CAD build for the part. Positions are in the model's coordinates, mm. A direction names the side the tool comes from. Give positions to 0.01 mm unless a question says otherwise; leave off trailing zeros. Loops run counter-clockwise (first coordinate to the right, second up) from the corner with the lowest first, then second, coordinate; pieces in that order, holes last.
```python
from build123d import *

# Parameters (mm, degrees)
F0_W     = 56
F0_H     = 50
F0_R     = 1.65
F0_R_2   = 23
F0_R_3   = 21.5
F1_DEPTH = 28
F2_R     = 21.5
F3_DEPTH = 25
F4_R     = 1.65
F5_DEPTH = 28.001
F7_DEPTH = 25
F6_R     = 23
F6_R_2   = 21.5
F8_DEPTH = 25


with BuildPart() as f1:
    # F0 (on Front) → F1 (new body)
    with BuildSketch(Plane.XZ):
        Rectangle(F0_W, F0_H)
        with Locations((23, -20)):
            Circle(F0_R, mode=Mode.SUBTRACT)
        with Locations((-23, 20)):
            Circle(F0_R, mode=Mode.SUBTRACT)
        Circle(F0_R_2, mode=Mode.SUBTRACT)
        Circle(F0_R_2)
        Circle(F0_R_3, mode=Mode.SUBTRACT)
        Circle(F0_R_3)
        with Locations((23, -20)):
            Circle(F0_R)
        with Locations((-23, 20)):
            Circle(F0_R)
    extrude(amount=F1_DEPTH)

    # F2 (on face) → F3 (cut)
    with BuildSketch(Plane.XZ.offset(28)):
        Circle(F2_R)
    extrude(amount=-F3_DEPTH, mode=Mode.SUBTRACT)

    # F4 (on face) → F5 (cut, through all)
    with BuildSketch(Plane.XZ.offset(28)):
        with Locations((-23, 20)):
            Circle(F4_R)
        with Locations((23, -20)):
            Circle(F4_R)
    extrude(amount=-F5_DEPTH, mode=Mode.SUBTRACT)

    # F7 (cut): a face of the model
    f7_faces = [f1.faces().sort_by_distance(p)[0] for p in [
        (0, -28, -24.2492670248),
    ]]
    extrude(f7_faces, amount=-F7_DEPTH, mode=Mode.SUBTRACT)

    # F6 (on face) → F8 (join)
    with BuildSketch(Plane.XZ.offset(3)):
        Circle(F6_R)
        Circle(F6_R_2, mode=Mode.SUBTRACT)
    extrude(amount=F8_DEPTH)


solid = f1.part
```
1. Saw through at B-B, the plane y = -4. List the corners of the cut face in (x, z), and give its area (3 significant figures).
Responses:
outline: circle Ø46 at (0, 0); hole circle Ø43 at (0, 0)
area: 210 mm2
2. Probe line 1 along Z through (x, y) = (0, -8.25); line 2 along Z through (x, y) = (23, -0.85); line 3 along Y through (x, z) = (2.5, -21). List the from-to ranges inside material, lowest first.
Responses:
line 1: z = -23 to -21.5, 21.5 to 23
line 2: z = -25 to -21.65, -18.35 to 25
line 3: y = -3 to 0
3. Saw through at D-D, the plane z = 8. List the corners of the cut face in (x, y), and give its area (3 significant figures).
Responses:
outline: (-28, -3) - (-21.56, -3) - (-21.56, -28) - (-19.96, -28) - (-19.96, -3) - (19.96, -3) - (19.96, -28) - (21.56, -28) - (21.56, -3) - (28, -3) - (28, 0) - (-28, 0) - close
area: 248 mm2
4. Drop flat-ended pins along their axis: pin 1 (1 mm diameter, centred on y = -18, z = -5, fed in from +X); pin 2 (2 mm diameter, centred on y = -18, z = 11.5, fed in from +X); pin 3 (4 mm diameter, centred on y = -10.5, z = -16.5, fed in from -X); pin 4 (3 mm diameter, centred on x = -23, z = 20, fed in from -Y). Give the stop position or say it passes through.
Responses:
pin 1: stops at x = 22.56
pin 2: stops at x = 20.46
pin 3: stops at x = -17.85
pin 4: passes through
5. Saw through at A-A, the plane x = 0. List the corners of the cut face in (y, z), and give its area (3 significant figures).
Responses:
outline: (-28, -23) - (-3, -23) - (-3, -25) - (0, -25) - (0, 25) - (-3, 25) - (-3, 23) - (-28, 23) - (-28, 21.5) - (-3, 21.5) - (-3, -21.5) - (-28, -21.5) - close
area: 225 mm2
6. Tool access for faces 1 (the face through (14, -28, -17)), 2 (the face through (-2.799, -15.325, 21.317)): list every direction of +Z, -Z, +X, -X, +Y, -Y with a clear straight run to the whole face (end or side of a thin tool).
Responses:
face 1: +Z, -Z, +X, -X, -Y
face 2: -Y
7. Pull direction Z, two halves, no side cores. Call faces 3 (the face through (-28, -1, 0)), 4 (the face through (21.784, -1.521, -18.885)), 5 (the face through (-2.994, -15.325, 22.804)): released by +Z, released by -Z, zero draft, split by the parting line, or undercut.
Responses:
face 3: zero draft
face 4: undercut
face 5: split by the parting line
8. Saw through at C-C, the plane z = -20. List the corners of the cut face in (x, y), and give its area (3 significant figures).
Responses:
outline: (-28, -3) - (-11.36, -3) - (-11.36, -28) - (-7.89, -28) - (-7.89, -3) - (7.89, -3) - (7.89, -28) - (11.36, -28) - (11.36, -3) - (21.35, -3) - (21.35, 0) - (-28, 0) - close; (24.65, -3) - (28, -3) - (28, 0) - (24.65, 0) - close
area: 331 mm2
